Input: part model. Units: mm. Frame: model coordinates. Face numbers are marked on the shaded views. A direction names the side the tool comes from. Coordinates: 2 decimals unless noted, no trailing zeros. Order: outer loops, then holes, each group sorted by start corner. A loop starts at its lowest first (then second) coordinate and runs counter-clockwise, first axis right, second up. Notation, with made-up numbers: (37, 6) -> (56, 6) arc R23 ccw to (56, 19) -> close; hole circle Ø4 at (65.25, 74.5). An arc over 180 degrees is marked (long way). One line per question, with ' | ' between items.
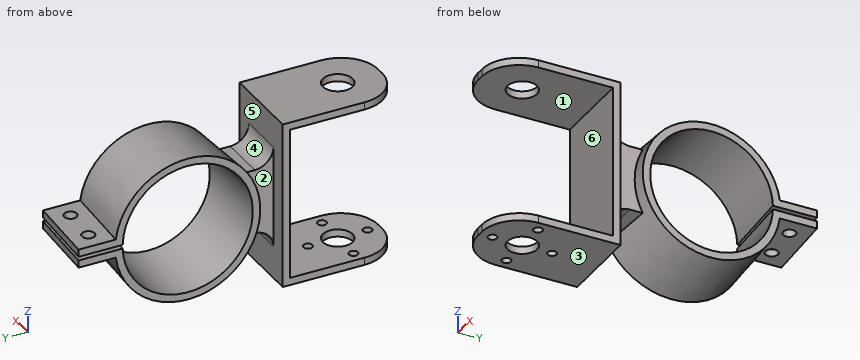
```python
from build123d import *

# Parameters (mm, degrees)
SKETCH3_R           = 1.7
CUT_EXTRUDE1_DEPTH  = 10
SKETCH4_W           = 22
SKETCH4_H           = 45
BOSS_EXTRUDE1_DEPTH = 2
BOSS_EXTRUDE3_REACH = 64.45
SKETCH6_W           = 12.5
SKETCH6_H           = 17.5
SKETCH7_W           = 22
SKETCH7_H           = 2
BOSS_EXTRUDE4_DEPTH = 30
SKETCH8_R           = 4
CUT_EXTRUDE2_DEPTH  = 76.59761901
SKETCH9_R           = 1.2
CUT_EXTRUDE3_DEPTH  = 30
FILLET1_R           = 10
FILLET2_R           = 5


with BuildPart() as part:
    # Sketch2 → Loft1 section 0
    with BuildSketch(Plane(origin=(20, 0, 0), x_dir=(0, 0, -1), z_dir=(1, 0, 0))):
        with BuildLine():
            Line((-2.5, 18.332586185), (-2.5, 28.332586185))
            Line((-2.5, 28.332586185), (-0.5, 28.332586185))
            Line((-0.5, 28.332586185), (-0.5, 16.492422502))
            ThreePointArc((-0.5, 16.492422502), (0, -16.5), (0.5, 16.492422502))
            Line((0.5, 16.492422502), (0.5, 28.332586185))
            Line((0.5, 28.332586185), (2.5, 28.332586185))
            Line((2.5, 28.332586185), (2.5, 18.332586185))
            ThreePointArc((2.5, 18.332586185), (0, -18.502262463), (-2.5, 18.332586185))
        make_face()
    # Sketch1 → Loft1 section 1
    with BuildSketch(Plane(origin=(0, 0, 0), x_dir=(0, 0, -1), z_dir=(1, 0, 0))):
        with BuildLine():
            Line((-2.5, 19.339079606), (-2.5, 29.339079606))
            Line((-2.5, 29.339079606), (-0.502358537, 29.339079606))
            Line((-0.502358537, 29.339079606), (-0.502358537, 17.492788111))
            ThreePointArc((-0.502358537, 17.492788111), (0, -17.5), (0.502358537, 17.492788111))
            Line((0.502358537, 17.492788111), (0.502358537, 29.339079606))
            Line((0.502358537, 29.339079606), (2.5, 29.339079606))
            Line((2.5, 29.339079606), (2.5, 19.339079606))
            ThreePointArc((2.5, 19.339079606), (0, -19.5), (-2.5, 19.339079606))
        make_face()
    loft()

    # Sketch3 → Cut-Extrude1 (cut)
    with BuildSketch(Plane(origin=(0, 0, -2.5), x_dir=(-1, 0, 0), z_dir=(0, 0, -1))):
        with Locations((-15, 23.577882113)):
            Circle(SKETCH3_R)
        with Locations((-5, 24.081128823)):
            Circle(SKETCH3_R)
    extrude(amount=-CUT_EXTRUDE1_DEPTH, mode=Mode.SUBTRACT)

    # Sketch6 → Boss-Extrude3 (add, up to next)
    with BuildSketch(Plane(origin=(0, -25, 0), x_dir=(1, 0, 0), z_dir=(0, 1, 0)), mode=Mode.PRIVATE) as boss_extrude3_sk1:
        with Locations((10, 0)):
            Rectangle(SKETCH6_W, SKETCH6_H)
    boss_extrude3_tool1 = extrude(boss_extrude3_sk1.sketch, amount=BOSS_EXTRUDE3_REACH, mode=Mode.PRIVATE) - part.part


with BuildPart() as body_2:
    # Sketch4 → Boss-Extrude1 (new body)
    with BuildSketch(Plane(origin=(0, -25, 0), x_dir=(1, 0, 0), z_dir=(0, 1, 0))):
        with Locations((10, 0)):
            Rectangle(SKETCH4_W, SKETCH4_H)
    extrude(amount=-BOSS_EXTRUDE1_DEPTH)


with BuildPart() as part_1:
    add(part.part)

    add(body_2.part)  # Boss-Extrude3 merges body 2
    add(boss_extrude3_tool1.solids().sort_by_distance((10, -25, 0))[0])

    # Sketch7 → Boss-Extrude4 (add)
    with BuildSketch(Plane.XZ.offset(27)):
        with Locations((10, 21.5)):
            Rectangle(SKETCH7_W, SKETCH7_H)
        with Locations((10, -21.5)):
            Rectangle(SKETCH7_W, SKETCH7_H)
    extrude(amount=BOSS_EXTRUDE4_DEPTH)

    # Sketch8 → Cut-Extrude2 (cut, through all)
    with BuildSketch(Plane.XY.offset(22.5)):
        with Locations(Location((10, -45.591327039, 0), (0, 0, 180))):
            Circle(SKETCH8_R)
    extrude(amount=-CUT_EXTRUDE2_DEPTH, mode=Mode.SUBTRACT)

    # Sketch9 → Cut-Extrude3 (cut)
    with BuildSketch(Plane(origin=(0, 0, -22.5), x_dir=(-1, 0, 0), z_dir=(0, 0, -1))):
        with Locations((-10, -37.591327039)):
            Circle(SKETCH9_R)
        with Locations((-2, -45.591327039)):
            Circle(SKETCH9_R)
        with Locations((-10, -53.591327039)):
            Circle(SKETCH9_R)
        with Locations((-18, -45.591327039)):
            Circle(SKETCH9_R)
    extrude(amount=-CUT_EXTRUDE3_DEPTH, mode=Mode.SUBTRACT)

    # Fillet1
    fillet1_edges = [part_1.edges().sort_by_distance(p)[0] for p in [
        (21, -57, -21.5),
        (-1, -57, 21.5),
        (21, -57, 21.5),
        (-1, -57, -21.5),
    ]]
    fillet(fillet1_edges, radius=FILLET1_R)

    # Fillet2
    fillet2_edges = [part_1.edges().sort_by_distance(p)[0] for p in [
        (10, -25, -8.75),
        (10, -25, 8.75),
    ]]
    fillet(fillet2_edges, radius=FILLET2_R)


solid = part_1.part
```
1. Pin query (flat end, axial travel): pin 1 Ø4 at (x, y) = (5, 24.08) entering from +Z; pin 2 Ø4 at (x, y) = (9.5, -18) entering from +Z; pin 3 Ø5 at (x, y) = (3.5, -17.5) entering from -Z. Return the tip coordinate at first contact, or that it passes through.
Recorded:
pin 1: stops at z = 2.5 | pin 2: stops at z = 10.3 | pin 3: stops at z = -12.19
2. Mould query, pull axis Z, two halves, no side actions, for the marked faces 1, 2 and 3. Classes: released by +Z, released by -Z, zero draft, split by the parting line, or undercut.
Recorded:
face 1: undercut | face 2: zero draft | face 3: released by -Z
3. Cut plane B-B, the plane x = 15. State how many separate pieces and enclosed holes the cut face has, and give its area (3 significant figures).
Recorded:
separate pieces: 3 | enclosed holes: 0 | area: 586 mm^2
4. Ray query, line 1 (Y direction, x = 10, z = -21.3); line 2 (Z direction, x = 1.25, y = -51); line 3 (Y direction, x = 14.5, z = 9.5). Return the intervals inside material, ascending. Write a range as [from, to].
Recorded:
line 1: y = [-57, -54.79], [-52.39, -49.59], [-41.59, -38.79], [-36.39, -25] | line 2: z = [-22.5, -20.5], [20.5, 22.5] | line 3: y = [-27, -22.63], [-16.2, -13.83], [13.83, 16.2]
5. Cut plane A-A, the plane y = -35. Return loops of the section in (x, z), and give its area (3 significant figures).
Recorded:
outline: (-1, -22.5) -> (21, -22.5) -> (21, -20.5) -> (-1, -20.5) -> close; (-1, 20.5) -> (21, 20.5) -> (21, 22.5) -> (-1, 22.5) -> close | area: 88.0 mm^2
6. Access query for the marked faces 4, 5 and 6. Directions: +Z, -Z, +X, -X, +Y, -Y. A direction counts if a zero-diameter tool reaches every point of the face in a straight line with its end or side. Return the directions, or none.
Recorded:
face 4: +Z, +X, -X | face 5: none | face 6: +X, -X, -Y
